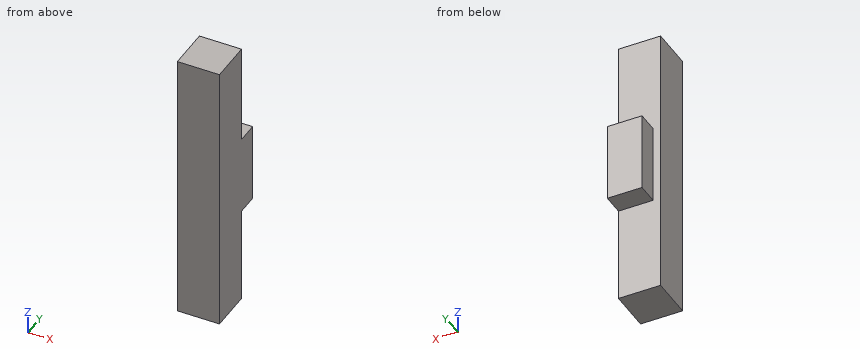
Autodesk Inventor part; units mm, degrees
ref_plane "YZ Plane" through (0, 0, 0) normal (1, 0, 0) x (0, 1, 0)
ref_plane "XZ Plane" through (0, 0, 0) normal (0, 1, 0) x (-1, 0, 0)
ref_plane "XY Plane" through (0, 0, 0) normal (0, 0, 1) x (1, 0, 0)
sketch "Sketch1" plane through (0, 0, 0) normal (0, 1, 0) x (-1, 0, 0)
  line L0 (0, 0) -> (50.8, 0)
  line L1 (50.8, 0) -> (50.8, -334)
  line L2 (50.8, -334) -> (0, -334)
  line L3 (0, -334) -> (0, 0)
  dimension "d0" = 50.8
  dimension "d1" = 334
extrude "Extrusion1" add sketch "Sketch1" along normal blind 77
sketch "Sketch3" plane through (0, 0, 0) normal (1, 0, 0) x (0, 0, -1)
  line L0 (0, 77) -> (121, 77)
  line L1 (121, 77) -> (121, 51.2)
  line L2 (121, 51.2) -> (0, 51.2)
  line L3 (0, 51.2) -> (0, 77)
  line L4 (0, 77) -> (334, 77)
  line L5 (334, 77) -> (217, 77)
  line L6 (217, 77) -> (217, 51.2)
  line L7 (217, 51.2) -> (334, 51.2)
  line L8 (334, 51.2) -> (334, 77)
  point P0 (0, 0)
  dimension "d9" = 25.8
  dimension "d10" = 117
  dimension "d11" = 25.8
  dimension "d17" = 96
extrude "Extrusion2" cut sketch "Sketch3" against normal blind 52.8
sketch "Sketch6" plane through (0, 77, 0) normal (0, 1, 0) x (1, 0, 0)
  line L0 (-50.8, 217) -> (-50.8, 121)
  line L1 (0, 217) -> (-50.8, 217)
  line L2 (-50.8, 121) -> (-41.8, 121)
  line L3 (-41.8, 121) -> (-41.8, 217)
  line L4 (-41.8, 217) -> (-50.8, 217)
  line L5 (-50.8, 217) -> (-50.8, 121)
  point P0 (0, 0)
  dimension "d18" = 9
extrude "Extrusion4" cut sketch "Sketch6" against normal blind 25.8
properties part number "PiezaPuerta-1"
Geometry: final body of the model. Coordinates: model frame, mm. Round coordinates to 2 decimals unless told otherwise and drop trailing zeros. Order: outer loops, then holes, each group sorted by start corner. A loop starts at its lowest first (then second) coordinate and runs counter-clockwise, first axis right, second up. Notation, with made-up numbers: (83.5, -14) - (89.5, -14) arc R16 cw to (89.5, 17) - close; hole circle Ø9 at (-20, 64.5). An arc over 180 degrees is marked (long way). Use CSV: the item, a comma, the result in double quotes. Start each with the question number.
Q1. Material intervals for line 1 along Y through (x, z) = (-20.5, -45.5); line 2 along Z through (x, y) = (-19, 60.5); line 3 along X through (y, z) = (69, -178), sorted ascending. Write a range as from..to.
Q2. Section query C-C (y = 57). Return loops of the section in (x, z), and give its area (3 significant figures).
Q3. First-contact query: pin 1 (5 mm diameter, centred on x = -25, z = -240, fed in from +Y); pin 2 (13 mm diameter, centred on y = 60.5, z = -163, fed in from -X); pin 3 (7.5 mm diameter, centred on x = -27, y = 65, fed in from +Z). Flat tips, straight axial feed; report the tip coordinate or a pass-through.
Q4. Section query B-B (z = -188). Return loops of the section in (x, y).
Q5. Section query D-D (z = -45). Return loops of the section in (x, y).
Q6. Section query A-A (x = -17). Return loops of the section in (y, z).
Result set:
1,line 1,"y = 0..51.2"
1,line 2,"z = -217..-121"
1,line 3,"x = -41.8..0"
2,outline,"(-41.8, -217) - (0, -217) - (0, -121) - (-41.8, -121) - close"
2,area,"4,010 mm2"
3,pin 1,"stops at y = 51.2"
3,pin 2,"stops at x = -41.8"
3,pin 3,"stops at z = -121"
4,outline,"(-50.8, 0) - (0, 0) - (0, 77) - (-41.8, 77) - (-41.8, 51.2) - (-50.8, 51.2) - close"
5,outline,"(-50.8, 0) - (0, 0) - (0, 51.2) - (-50.8, 51.2) - close"
6,outline,"(0, -334) - (51.2, -334) - (51.2, -217) - (77, -217) - (77, -121) - (51.2, -121) - (51.2, 0) - (0, 0) - close"
